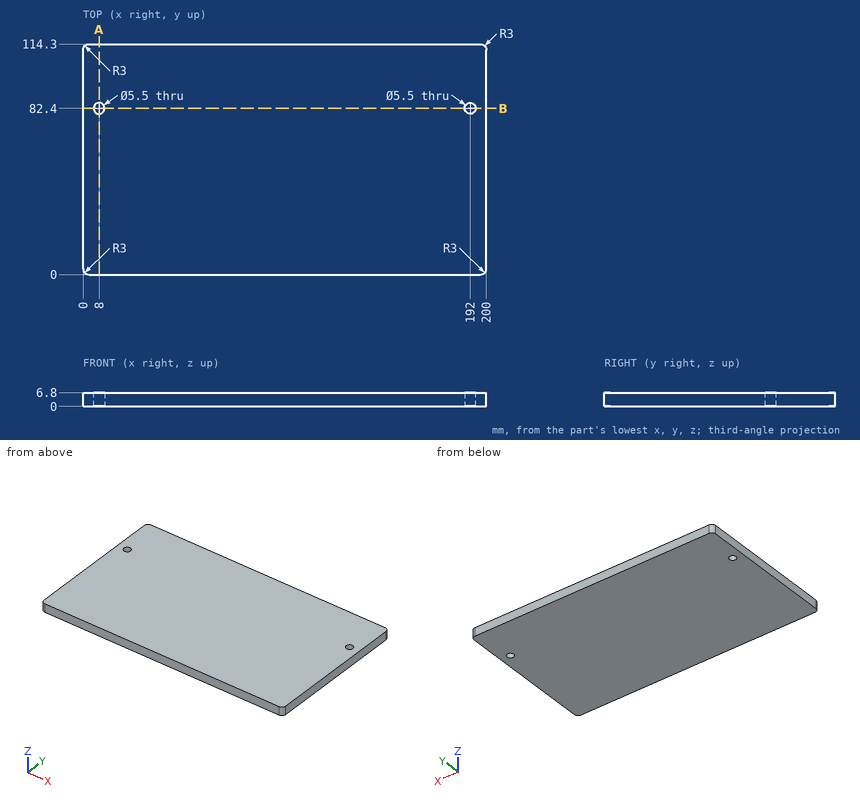
Source: three-view drawing plus pictorial views. Frame: mm from the lowest corner of the part. Round coordinates to 2 decimals unless told otherwise and drop trailing zeros. Order: outer loops, then holes, each group sorted by start corner. A loop starts at its lowest first (then second) coordinate and runs counter-clockwise, first axis right, second up. Notation, with made-up numbers: (42, 43) - (48, 43) arc R21 cw to (48, 51) - close; hole circle Ø4 at (37, 79). An arc over 180 degrees is marked (long way). Write each question's results on one line, items separated by ' | '.
Item 1: Section A-A, the plane x = 8. Return the cut outline in (y, z).
Completed:
outline: (0, 0) - (79.65, 0) - (79.65, 6.8) - (0, 6.8) - close; (85.15, 0) - (114.3, 0) - (114.3, 6.8) - (85.15, 6.8) - close
Item 2: First-contact query: pin 1 Ø5 at (x, y) = (8, 82.4) entering from -Z. Flat tip, straight axial feed; report the tip coordinate or a pass-through.
Completed:
pin 1: through
Item 3: Section B-B, the plane y = 82.4. Return the cut outline in (x, z).
Completed:
outline: (0, 0) - (5.25, 0) - (5.25, 6.8) - (0, 6.8) - close; (10.75, 0) - (189.25, 0) - (189.25, 6.8) - (10.75, 6.8) - close; (194.75, 0) - (200, 0) - (200, 6.8) - (194.75, 6.8) - close
Item 4: Material intervals for line 1 along X through (y, z) = (82.4, 4.5); line 2 along Y through (x, z) = (192, 1.5), sorted ascending. Write a range as [from, to].
Completed:
line 1: [0, 5.25], [10.75, 189.25], [194.75, 200] | line 2: [0, 79.65], [85.15, 114.3]
